from build123d import *

# Parameters (mm, degrees)
SKETCH1_R                = 10
BOSS_EXTRUDE1_DEPTH      = 47
SHELL1_T                 = -2
SKETCH2_W                = 8
SKETCH2_H                = 17
CUT_EXTRUDE1_DEPTH       = 45
SKETCH3_R                = 2.625
CUT_EXTRUDE2_DEPTH       = 50.081564767
SKETCH4_R                = 13.75
BOSS_EXTRUDE2_DEPTH      = 22
BOSS_EXTRUDE3_START      = 20
SKETCH5_R                = 13.75
SKETCH5_R_2              = 12.75
BOSS_EXTRUDE3_DEPTH      = 20
FILLET1_R                = 0.5
SKETCH6_W                = 8
SKETCH6_H                = 30
CUT_EXTRUDE3_DEPTH       = 10
FILLET2_R                = 4
REVOLVE5_ANGLE           = 4
FILLET3_R                = 1
CIRPATTERN1_COUNT        = 4
FILLET3_OF_CIRPATTERN1_R = 1
SKETCH9_R                = 11.75
CUT_EXTRUDE4_DEPTH       = 15
CUT_EXTRUDE6_DEPTH       = 74.724950074
CUT_EXTRUDE6_DEPTH_BACK  = 74.724950074
SKETCH10_R               = 2.625
SKETCH11_W               = 15
SKETCH11_H               = 2
CUT_EXTRUDE7_DEPTH       = 15
FILLET4_R                = 2


# Some blends are built 0.0001 mm under size
with BuildPart() as part:
    # Sketch1 → Boss-Extrude1 (new body)
    with BuildSketch(Plane(origin=(0, 0, 0), x_dir=(1, 0, 0), z_dir=(0, 1, 0))):
        with Locations(Location((0, 0, 0), (0, 0, 270))):
            Circle(SKETCH1_R)
    extrude(amount=BOSS_EXTRUDE1_DEPTH)

    # Shell1
    shell1_openings = [part.faces().sort_by_distance(p)[0] for p in [
        (0, 47, 0),
    ]]
    offset(amount=SHELL1_T, openings=shell1_openings, kind=Kind.INTERSECTION)

    # Sketch2 → Cut-Extrude1 (cut)
    with BuildSketch(Plane(origin=(0, 47, 0), x_dir=(1, 0, 0), z_dir=(0, 1, 0))):
        Rectangle(SKETCH2_W, SKETCH2_H)
    extrude(amount=-CUT_EXTRUDE1_DEPTH, mode=Mode.SUBTRACT)

    # Sketch3 → Cut-Extrude2 (cut, through all)
    with BuildSketch(Plane.XY):
        with Locations(Location((0, 7, 0), (0, 0, 90))):
            Circle(SKETCH3_R)
    extrude(amount=-CUT_EXTRUDE2_DEPTH, mode=Mode.SUBTRACT)

    # Sketch4 → Boss-Extrude2 (add)
    with BuildSketch(Plane(origin=(0, 47, 0), x_dir=(1, 0, 0), z_dir=(0, 1, 0))):
        with Locations(Location((0, 0, 0), (0, 0, 270))):
            Circle(SKETCH4_R)
    extrude(amount=BOSS_EXTRUDE2_DEPTH)

    # Sketch5 → Boss-Extrude3 (add)
    with BuildSketch(Plane.XZ.offset(-47).offset(BOSS_EXTRUDE3_START)):
        with Locations(Location((0, 0, 0), (0, 0, 270))):
            Circle(SKETCH5_R)
        with Locations(Location((0, 0, 0), (0, 0, 270))):
            Circle(SKETCH5_R_2, mode=Mode.SUBTRACT)
    extrude(amount=-BOSS_EXTRUDE3_DEPTH)

    # Fillet1
    fillet1_edges = [part.edges().sort_by_distance(p)[0] for p in [
        (0, 47, -10),
        (0, 47, 12.75),
    ]]
    fillet(fillet1_edges, radius=FILLET1_R)

    # Sketch6 → Cut-Extrude3 (cut)
    with BuildSketch(Plane(origin=(0, 0, 0), x_dir=(0, 0, -1), z_dir=(1, 0, 0))):
        with Locations((0, 19.375)):
            Rectangle(SKETCH6_W, SKETCH6_H)
    extrude(amount=-CUT_EXTRUDE3_DEPTH, mode=Mode.SUBTRACT)

    # Fillet2
    fillet2_edges = [part.edges().sort_by_distance(p)[0] for p in [
        (-8.04667731, 4.375, 4),
        (-8.04667731, 4.375, -4),
    ]]
    fillet(fillet2_edges, radius=FILLET2_R - 0.0001)  # a hair under: the kernel refuses the full size

    # Sketch8 → Revolve5 (revolve, symmetric)
    with BuildSketch(Plane(origin=(0, 0, 0), x_dir=(0, 0, -1), z_dir=(1, 0, 0))) as revolve5_sk:
        Polygon((13.75, 27), (18.75, 27), (13.75, 42), align=None)
    revolve5 = revolve(axis=Axis((0, 88.2, 0), (0, -1, 0)), revolution_arc=REVOLVE5_ANGLE / 2)
    revolve5 = revolve5 + revolve(revolve5_sk.sketch, axis=Axis((0, 88.2, 0), (0, 1, 0)), revolution_arc=REVOLVE5_ANGLE / 2)

    # Fillet3
    fillet3_edges = [part.edges().sort_by_distance(p)[0] for p in [
        (0, 27, -18.75),
    ]]
    fillet(fillet3_edges, radius=FILLET3_R)

    # CirPattern1: Revolve5 ×4 about axis
    cirpattern1_axis = Axis((0, 88.2, 0), (0, -1, 0))
    for i in range(1, CIRPATTERN1_COUNT):
        add(revolve5.rotate(cirpattern1_axis, i * 360 / CIRPATTERN1_COUNT))

    # Fillet3 of CirPattern1
    fillet3_of_cirpattern1_edges = [part.edges().sort_by_distance(p)[0] for p in [
        (18.75, 27, 0),
        (0, 27, 18.75),
        (-18.75, 27, 0),
    ]]
    fillet(fillet3_of_cirpattern1_edges, radius=FILLET3_OF_CIRPATTERN1_R)

    # Sketch9 → Cut-Extrude4 (cut)
    with BuildSketch(Plane(origin=(0, 69, 0), x_dir=(1, 0, 0), z_dir=(0, 1, 0))):
        with Locations(Location((0, 0, 0), (0, 0, 270))):
            Circle(SKETCH9_R)
    extrude(amount=-CUT_EXTRUDE4_DEPTH, mode=Mode.SUBTRACT)

    # Sketch10 → Cut-Extrude6 (cut, two sides: drawn at the far end of the back side and taken through both)
    with BuildSketch(Plane.XY.offset(-CUT_EXTRUDE6_DEPTH_BACK)):
        with Locations((0, 59)):
            Circle(SKETCH10_R)
    extrude(amount=CUT_EXTRUDE6_DEPTH + CUT_EXTRUDE6_DEPTH_BACK, mode=Mode.SUBTRACT)

    # Sketch11 → Cut-Extrude7 (cut)
    with BuildSketch(Plane(origin=(0, 69, 0), x_dir=(1, 0, 0), z_dir=(0, 1, 0))):
        with Locations((0, -13.5)):
            Rectangle(SKETCH11_W, SKETCH11_H)
    cut_extrude7 = extrude(amount=-CUT_EXTRUDE7_DEPTH, mode=Mode.SUBTRACT)

    # Mirror1: Cut-Extrude7 across plane
    add(cut_extrude7.mirror(Plane.XY), mode=Mode.SUBTRACT)

    # Fillet4
    # the kernel refuses this fillet: 2 mm, written as the material it adds along each edge
    with BuildSketch(Plane(origin=(-10.728219619, 54, -12.5), x_dir=(0, 1, 0), z_dir=(1, 0, 0))) as fillet4_piece_1_section:
        with BuildLine():
            CenterArc((FILLET4_R, -FILLET4_R), FILLET4_R, 90, 90)
            Line((0, -FILLET4_R), (0, 0))
            Line((0, 0), (FILLET4_R, 0))
        make_face()
    fillet4_piece_1 = extrude(amount=21.456439237, mode=Mode.PRIVATE)
    fillet4_piece_1 = fillet4_piece_1 & Plane(origin=(0, 54.536479762, 0), x_dir=(0, 0, 1), z_dir=(0, -1, 0)) * Cylinder(13.75, 51, mode=Mode.PRIVATE)
    add(fillet4_piece_1)
    with BuildSketch(Plane(origin=(-10.728219619, 54, 12.5), x_dir=(0, 0, 1), z_dir=(1, 0, 0))) as fillet4_piece_2_section:
        with BuildLine():
            CenterArc((FILLET4_R, -FILLET4_R), FILLET4_R, 90, 90)
            Line((0, -FILLET4_R), (0, 0))
            Line((0, 0), (FILLET4_R, 0))
        make_face()
    fillet4_piece_2 = extrude(amount=21.456439237, mode=Mode.PRIVATE)
    fillet4_piece_2 = fillet4_piece_2 & Plane(origin=(0, 54.536497639, 0), x_dir=(0, 0, 1), z_dir=(0, -1, 0)) * Cylinder(13.75, 51, mode=Mode.PRIVATE)
    add(fillet4_piece_2)


solid = part.part
Input: part model. Units: mm. Frame: model coordinates. A direction names the side the tool comes from. Coordinates: 2 decimals unless noted, no trailing zeros. Write each loop counter-clockwise with the first axis right and the second up, starting at its lowest first coordinate (ties: lowest second). Pieces come first, ordered by that corner, then holes. Notation, with made-up numbers: M 33.25,5.5 L 83.25,5.5 A19 cw 83.25,28.5 Z; hole C 49,83 d11. An arc over 180 degrees is marked long. Answer as a JSON object with one key per item and string values. Group by question number.
(1) Section C-C on y = 21.5. Output: boundary loops of the cut face in (x, z).
(2) Section D-D on y = 7. Output: boundary loops of the cut face in (x, z) (3 decimals).
(3) Section A-A on y = 59. Output: boundary loops of the cut face in (x, z) (3 decimals).
(4) Section B-B on y = 38. Output: boundary loops of the cut face in (x, z).
(5) Mould query, pull axis Y, two halves, no side actions, for faces 1 (the face through (0.01, 35.25, 16)), 2 (the face through (-8.49, 5.52, 2.8)), 3 (the face through (-5, 27, -12)). Classes: pulls with the +Y half, pulls with the -Y half, needs draft (parallel to the pull), parting line crosses it, or undercut.
(6) Contact query for flat-ended pins moving along their axis: P1, Ø2, axis at x = 0.5, z = 2, coming from the +Y side; P2, Ø4, axis at y = 43.5, z = -13.5, coming from the -X side; P3, Ø6.5, axis at x = -1.5, y = 21, coming from the -Z side. Output: stop coordinate, or through.
(7) Set-up query: faces 4 (the face through (0, 54, 0)), 5 (the face through (-4, 25, 8)), 6 (the face through (-0.08, 55.125, -12.702)). Return all of +Z, -Z, +X, -X, +Y, -Y with unobstructed straight access to the full face (end or side cutting, diameter ignored); none if empty.
(8) Ray query, line 1 along Z through (x, y) = (-8.5, 35); line 2 along Z through (x, y) = (9, 32.5); line 3 along Y through (x, z) = (-3, 2). Return the intervals inside material, ascending. Write a range as [from, to].
Result set:
{
 "1": {"outline": "M -9.17,-4 A10 ccw long -9.17,4 L -6.93,4 A8 cw -4,6.93 L -4,8.5 L 4,8.5 L 4,6.93 A8 cw 4,-6.93 L 4,-8.5 L -4,-8.5 L -4,-6.93 A8 cw -6.93,-4 Z"},
 "2": {"outline": "M -9.268,-3.756 A10 ccw -2.625,-9.649 L -2.625,-8.5 L -4,-8.5 L -4,-6.928 A8 cw -7.063,-3.756 Z; M -9.268,3.756 L -7.063,3.756 A8 cw -4,6.928 L -4,8.5 L 4,8.5 L 4,6.928 A8 cw 4,-6.928 L 4,-8.5 L 2.625,-8.5 L 2.625,-9.649 A10 ccw long Z"},
 "3": {"outline": "M -5.728,-12.5 L -2.625,-12.5 L -2.625,-11.453 A11.75 cw -2.625,11.453 L -2.625,12.5 L -5.728,12.5 A13.75 ccw Z; M 2.625,-12.5 L 5.728,-12.5 A13.75 ccw 5.728,12.5 L 2.625,12.5 L 2.625,11.453 A11.75 cw 2.625,-11.453 Z"},
 "4": {"outline": "M -15.07,-0.53 L -13.74,-0.48 A13.75 ccw -0.48,-13.74 L -0.53,-15.07 A15.08 ccw 0.53,-15.07 L 0.48,-13.74 A13.75 ccw 13.74,-0.48 L 15.07,-0.53 A15.08 ccw 15.07,0.53 L 13.74,0.48 A13.75 ccw 0.48,13.74 L 0.53,15.07 A15.08 ccw -0.53,15.07 L -0.48,13.74 A13.75 ccw -13.74,0.48 L -15.07,0.53 A15.08 ccw Z; C 0,0 d20; hole C 0,0 d25.5; hole M -4,-8.5 L 4,-8.5 L 4,-6.93 A8 ccw 4,6.93 L 4,8.5 L -4,8.5 L -4,6.93 A8 ccw -4,-6.93 Z"},
 "5": {"face 1": "pulls with the +Y half", "face 2": "undercut", "face 3": "pulls with the -Y half"},
 "6": {"P1": "stops at y = 54", "P2": "stops at x = -7.54", "P3": "stops at z = -10"},
 "7": {"face 4": "+Y", "face 5": "none", "face 6": "-Z, +X, -X, +Y"},
 "8": {"line 1": "z = [-10.81, -9.5], [-5.27, 5.27], [9.5, 10.81]", "line 2": "z = [-10.4, -9.03], [-4.36, 4.36], [9.03, 10.4]", "line 3": "y = [0, 2], [47, 54]"}
}
